from build123d import *

# Parameters (mm, degrees)
SALIENTE_EXTRUIR1_DEPTH = 10
SALIENTE_EXTRUIR2_DEPTH = 90
SALIENTE_EXTRUIR3_DEPTH = 50
CROQUIS6_W              = 56.928573576
CROQUIS6_H              = 55.923287038
CORTAR_EXTRUIR2_DEPTH   = 30
CROQUIS5_W              = 40
CROQUIS5_H              = 10
CROQUIS5_W_2            = 10
CROQUIS5_H_2            = 40
CORTAR_EXTRUIR1_DEPTH   = 5.7
CROQUIS7_R              = 2.5
CORTAR_EXTRUIR3_DEPTH   = 11
SKETCH1_W               = 156.521822712
SKETCH1_H               = 40.193765496
CUT_EXTRUDE1_DEPTH      = 40


with BuildPart() as part:
    # Croquis1 → Saliente-Extruir1 (new body)
    with BuildSketch(Plane(origin=(0, 0, 0), x_dir=(1, 0, 0), z_dir=(0, 1, 0))):
        Polygon((25, 20), (-65, 20), (-65, -20), (-15, -20), (-15, -70), (25, -70), (25, -20), align=None)
    extrude(amount=SALIENTE_EXTRUIR1_DEPTH)

    # Croquis2 → Saliente-Extruir2 (add, through all)
    with BuildSketch(Plane.XY.offset(70)):
        Polygon((12.2, 9.987376579), (12.2, 15.7), (17.8, 15.7), (17.8, 9.987376579), (15, 9.987376579), align=None)
        Polygon((-7.8, 9.987376579), (-7.8, 15.7), (-2.2, 15.7), (-2.2, 9.987376579), (-5, 9.987376579), align=None)
    extrude(amount=-SALIENTE_EXTRUIR2_DEPTH)

    # Croquis3 → Saliente-Extruir3 (add)
    with BuildSketch(Plane.ZY.offset(65)):
        Polygon((7.2, 10), (7.2, 15.7), (12.8, 15.7), (12.8, 10), (10, 10), align=None)
        Polygon((-12.8, 10), (-12.8, 15.7), (-7.2, 15.7), (-7.2, 10), (-10, 10), align=None)
    extrude(amount=-SALIENTE_EXTRUIR3_DEPTH)

    # Croquis6 → Cortar-Extruir2 (cut)
    with BuildSketch(Plane.ZY.offset(65)):
        Rectangle(CROQUIS6_W, CROQUIS6_H)
    extrude(amount=-CORTAR_EXTRUIR2_DEPTH, mode=Mode.SUBTRACT)

    # Croquis5 → Cortar-Extruir1 (cut)
    with BuildSketch(Plane(origin=(0, 15.7, 0), x_dir=(1, 0, 0), z_dir=(0, 1, 0))):
        with Locations((5, -65)):
            Rectangle(CROQUIS5_W, CROQUIS5_H)
        with Locations((5, 15)):
            Rectangle(CROQUIS5_W, CROQUIS5_H)
        with Locations((-30, 0)):
            Rectangle(CROQUIS5_W_2, CROQUIS5_H_2)
    extrude(amount=-CORTAR_EXTRUIR1_DEPTH, mode=Mode.SUBTRACT)

    # Croquis7 → Cortar-Extruir3 (cut, through all)
    with BuildSketch(Plane(origin=(0, 10, 0), x_dir=(1, 0, 0), z_dir=(0, 1, 0))):
        with Locations((-29, 10)):
            Circle(CROQUIS7_R)
        with Locations((-29, -10)):
            Circle(CROQUIS7_R)
        with Locations((15, 14)):
            Circle(CROQUIS7_R)
        with Locations((-5, 14)):
            Circle(CROQUIS7_R)
        with Locations((-5, -64)):
            Circle(CROQUIS7_R)
        with Locations((15, -64)):
            Circle(CROQUIS7_R)
    extrude(amount=-CORTAR_EXTRUIR3_DEPTH, mode=Mode.SUBTRACT)

    # Mirror1: part across plane


with BuildPart() as part_1:
    add(part.part)
    add(part.part.mirror(Plane.ZY.offset(35)))

    # Sketch1 → Cut-Extrude1 (cut)
    with BuildSketch(Plane(origin=(25, 0, 0), x_dir=(0, 0, -1), z_dir=(1, 0, 0))):
        Rectangle(SKETCH1_W, SKETCH1_H)
    extrude(amount=-CUT_EXTRUDE1_DEPTH, mode=Mode.SUBTRACT)


solid = part_1.part
Design review of the part built by this model. Coordinates are the model's own, in mm. A direction names the side the tool comes from. Give positions to 0.01 mm unless a question says otherwise; leave off trailing zeros. Loops run counter-clockwise (first coordinate to the right, second up) from the corner with the lowest first, then second, coordinate; pieces in that order, holes last. Notation, with made-up numbers: M 44.5,66 L 62.5,66 A16 cw 62.5,73 Z; hole C -26,-34.5 d10. An arc over 180 degrees is marked long. One line per question, with ' | ' between items. Start each with the question number.
1. Add section D-D (y = 4.5). Give the number of separate pieces and of enclosed holes in the cut face, plus the area to 3 significant figures.
2. Insertion check: P1, Ø1.7, axis at x = -19.5, y = 13.5, coming from the -Z side; P2, Ø1, axis at y = 10, z = 28, coming from the +X side; P3, Ø1.7, axis at x = -85.5, y = 12.5, coming from the -Z side; P4, Ø4.5, axis at x = -29, z = -10, coming from the +Y side. Each pin has a flat end and moves straight along its axis. Give the tip position at first contact, or say it passes through.
3. Add section B-B (y = 12.5). Write out the cut boundary in (x, z).
4. For faces 1 (the face through (-65, 13, 60)), 2 (the face through (-45, 13, 10)), 3 (the face through (-50, 13, -12.8)), 4 (the face through (-20, 13, -7.2)), 5 (the face through (-85, 13, -10)), list the 3-axis set-ups (+Z, -Z, +X, -X, +Y, -Y) from which the entire face can be reached by the end or side of a thin tool; tool diameter is ignored.
5. Add section A-A (z = 64). Write out the cut boundary in (x, y).
6. Add section C-C (x = -85). Write out the cut boundary in (y, z).
7. The part is to be moulded in two halves that separate along X. For faces 6 (the face through (-67.385, 5.07, 63.249)), 7 (the face through (-55, 5, 45)), 8 (the face through (-20, 13, -12.8)), say which applies: released by +X, released by -X, zero draft, split by the parting line, or undercut.
8. To check wall thickness, follow L1, parallel to Z at x = -29, y = 2.5; L2, parallel to Z at x = -65, y = 6.25; L3, parallel to X at y = 11.5, z = 11. State the ranges of each line that lie inside material, in increasing order.
Worked out:
1) separate pieces: 1 | enclosed holes: 8 | area: 5,040 mm²
2) P1: stops at z = -12.8 | P2: stops at x = -55 | P3: stops at z = -10 | P4: passes through
3) outline: M -87.8,-10 L -82.2,-10 L -82.2,60 L -87.8,60 Z; M -67.8,-10 L -62.2,-10 L -62.2,60 L -67.8,60 Z; M -55,-12.8 L -45,-12.8 L -45,-7.2 L -55,-7.2 Z; M -55,7.2 L -45,7.2 L -45,12.8 L -55,12.8 Z; M -25,-12.8 L -15,-12.8 L -15,-7.2 L -25,-7.2 Z; M -25,7.2 L -15,7.2 L -15,12.8 L -25,12.8 Z
4) face 1: +Z, +X, -X, +Y | face 2: +Z, -Z, +Y | face 3: -Z, +X, -X, +Y | face 4: +X, +Y | face 5: -Z, -X, +Y
5) outline: M -95,0 L -87.5,0 L -87.5,10 L -95,10 Z; M -82.5,0 L -67.5,0 L -67.5,10 L -82.5,10 Z; M -62.5,0 L -55,0 L -55,10 L -62.5,10 Z
6) outline: M 0,-20 L 10,-20 L 10,-16.5 L 0,-16.5 Z; M 0,-11.5 L 10,-11.5 L 10,-10 L 15.7,-10 L 15.7,60 L 10,60 L 10,61.5 L 0,61.5 Z; M 0,66.5 L 10,66.5 L 10,70 L 0,70 Z
7) face 6: undercut | face 7: released by +X | face 8: zero draft
8) L1: z = -20 to -12.5, -7.5 to 7.5, 12.5 to 20 | L2: z = -20 to -16.5, -11.5 to 61.5, 66.5 to 70 | L3: x = -87.8 to -82.2, -67.8 to -62.2, -55 to -45, -25 to -15
